The model under review builds one solid part; all positions refer to its coordinate system, in mm. A direction names the side the tool comes from. Round coordinates to 2 decimals unless told otherwise and drop trailing zeros. Write each loop counter-clockwise with the first axis right and the second up, starting at its lowest first coordinate (ties: lowest second). Pieces come first, ordered by that corner, then holes. Notation, with made-up numbers: (88, -10.5) - (132, -10.5) arc R21 cw to (132, 16.5) - close; hole circle Ø8 at (36.25, 88.5). An arc over 180 degrees is marked (long way). Use one line per item in the form item = value.
from build123d import *

# Parameters (mm, degrees)
SKETCH_1_R          = 10
SKETCH_1_R_2        = 4
EXTRUDE_1_DEPTH     = 35
CHAMFER_1_SIZE      = 1
SKETCH_3_W          = 15
SKETCH_3_H          = 20
CUT_EXTRUDE_1_DEPTH = 7.5
SKETCH_3_4_R        = 1.5
CUT_EXTRUDE_2_DEPTH = 42.533119315


with BuildPart() as part:
    # Sketch 1 → Extrude 1 (new body)
    with BuildSketch(Plane(origin=(0, 0, 0), x_dir=(0, 0, -1), z_dir=(1, 0, 0))):
        Circle(SKETCH_1_R)
        Circle(SKETCH_1_R_2, mode=Mode.SUBTRACT)
    extrude(amount=EXTRUDE_1_DEPTH)

    # Chamfer 1
    chamfer_1_edges = [part.edges().sort_by_distance(p)[0] for p in [
        (0, 0, 10),
        (35, 0, 10),
    ]]
    chamfer(chamfer_1_edges, length=CHAMFER_1_SIZE)

    # Sketch 3 → Cut-Extrude 1 (cut)
    with BuildSketch(Plane(origin=(0, -10, 0), x_dir=(-1, 0, 0), z_dir=(0, -1, 0))):
        with Locations((-7.5, 0)):
            Rectangle(SKETCH_3_W, SKETCH_3_H)
        with Locations((-27.5, 0)):
            Rectangle(SKETCH_3_W, SKETCH_3_H)
    extrude(amount=-CUT_EXTRUDE_1_DEPTH, mode=Mode.SUBTRACT)

    # Sketch 3_4 → Cut-Extrude 2 (cut, through all)
    with BuildSketch(Plane(origin=(0, -10, 0), x_dir=(-1, 0, 0), z_dir=(0, -1, 0))):
        with Locations(Location((-31, 6.5, 0), (0, 0, 90))):
            Circle(SKETCH_3_4_R)
        with Locations(Location((-24, 6.5, 0), (0, 0, 90))):
            Circle(SKETCH_3_4_R)
        with Locations(Location((-31, -6.5, 0), (0, 0, 90))):
            Circle(SKETCH_3_4_R)
        with Locations(Location((-24, -6.5, 0), (0, 0, 90))):
            Circle(SKETCH_3_4_R)
        with Locations(Location((-4, 6.5, 0), (0, 0, 90))):
            Circle(SKETCH_3_4_R)
        with Locations(Location((-11, 6.5, 0), (0, 0, 90))):
            Circle(SKETCH_3_4_R)
        with Locations(Location((-11, -6.5, 0), (0, 0, 90))):
            Circle(SKETCH_3_4_R)
        with Locations(Location((-4, -6.5, 0), (0, 0, 90))):
            Circle(SKETCH_3_4_R)
    extrude(amount=-CUT_EXTRUDE_2_DEPTH, mode=Mode.SUBTRACT)


solid = part.part
(1) Add section B-B on x = 11. Write out the cut boundary in (y, z), then the cut area to 3 significant figures.
Geometry results:
outline = (-2.5, -9.68) arc R10 ccw to (6, -8) - (-2.5, -8) - close; (-2.5, -5) - (8.66, -5) arc R10 ccw to (8.66, 5) - (-2.5, 5) - (-2.5, 3.12) arc R4 cw (long way) to (-2.5, -3.12) - close; (-2.5, 8) - (6, 8) arc R10 ccw to (-2.5, 9.68) - close
area = 103 mm2
(2) Add section A-A on y = 0. Count the separate pieces of the cut face and the enclosed holes in it, then the cut area to 3 significant figures.
Geometry results:
separate_pieces = 2
enclosed_holes = 8
area = 361 mm2
(3) To check wall thickness, follow L1, parallel to X at y = 1, z = 6.5; L2, parallel to Z at x = 17, y = -0.25; L3, parallel to X at y = 6, z = -7. State the ranges of each line that lie inside material, in increasing order.
Geometry results:
L1 = 0 to 2.5, 5.5 to 9.5, 12.5 to 22.5, 25.5 to 29.5, 32.5 to 35
L2 = -10 to -3.99, 3.99 to 10
L3 = 0.22 to 2.59, 5.41 to 9.59, 12.41 to 22.59, 25.41 to 29.59, 32.41 to 34.78
(4) Add section D-D on x = 16.5. Write out the cut boundary in (y, z), then the cut area to 3 significant figures.
Geometry results:
outline = circle Ø20 at (0, 0); hole circle Ø8 at (0, 0)
area = 264 mm2
(5) Insertion check: P1, Ø2, axis at x = 29.5, z = -7.5, coming from the -Y side; P2, Ø4, axis at y = 5.5, z = 5.5, coming from the -X side; P3, Ø4, axis at y = -6, z = 2, coming from the +X side; P4, Ø1, axis at y = -6.5, z = 2, coming from the -X side. Each pin has a flat end and moves straight along its axis. Give the tip position at first contact, or say it passes through.
Geometry results:
P1 = -2.5
P2 = 0
P3 = 20
P4 = 15
(6) Add section C-C on z = 0. Write out the cut boundary in (x, y).
Geometry results:
outline = (0, 4) - (35, 4) - (35, 9) - (34, 10) - (1, 10) - (0, 9) - close; (15, -10) - (20, -10) - (20, -4) - (15, -4) - close
(7) Machinability: for faces 1 (the flat face through (8, -2.5, -6)), 2 (the flat face through (20, -5, 0)), 3 (the cylindrical face through (31, 3, 5)), which of the approach directions +Z, -Z, +X, -X, +Y, -Y give a long, thin tool a straight path to every point of the face, cutting with its end or side? Answer none if there is none.
Geometry results:
face_1 = +Z, -Z, -X, -Y
face_2 = +Z, -Z, +X, -Y
face_3 = +Y, -Y
(8) The part is to be moulded in two halves that separate along Z. For faces 4 (the flat face through (35, 5, 0)), 5 (the cylindrical face through (24, 3, -5)), 6 (the conical face through (0.2, 9.2, -0.2)), say which applies: +Z half, -Z half, draft (parallel to the pull), parting line (faces both ways), or undercut.
Geometry results:
face_4 = draft
face_5 = undercut
face_6 = parting line
